from build123d import *

# Parameters (mm, degrees)
SKETCH_1_W          = 69.038205547
SKETCH_1_H          = 75.629640719
EXTRUDE_1_DEPTH     = 10
CUT_EXTRUDE_1_DEPTH = 103.8888545
FILLET_1_R          = 2
SHELL_START         = 2
SHELL_1_DEPTH       = 65.038205547
SKETCH_3_W          = 9
SKETCH_3_H          = 9
CUT_EXTRUDE_2_DEPTH = 103.887957646


# Read off the part's stored shape, not the designer's step: 쉘1
with BuildPart() as part:
    # 스케치1 → 보스-돌출1 (new body)
    with BuildSketch(Plane.XY):
        with Locations((34.519102774, 37.81482036)):
            Rectangle(SKETCH_1_W, SKETCH_1_H)
    extrude(amount=EXTRUDE_1_DEPTH)

    # 스케치2 → 컷-돌출1 (cut, through all)
    with BuildSketch(Plane(origin=(69.038205547, 0, 0), x_dir=(0, 0, -1), z_dir=(1, 0, 0))):
        with BuildLine():
            Line((-10, 75.629640719), (-10, 0))
            add(Edge.make_bspline(
                [(-5.96238454, 75.629640719), (-9.875617916, 37.91260995), (-10, 0)],
                knots=[0, 0, 0, 1, 1, 1], degree=2))
            Line((-5.96238454, 75.629640719), (-10, 75.629640719))
        make_face()
    extrude(amount=-CUT_EXTRUDE_1_DEPTH, mode=Mode.SUBTRACT)

    # 필렛1
    fillet_1_edges = [part.edges().sort_by_distance(p)[0] for p in [
        (69.038205547, 37.865383105, 8.928316045),
        (34.519102774, 75.629640719, 5.96238454),
        (0, 37.865383105, 8.928316045),
        (34.519102774, 0, 10),
    ]]
    fillet(fillet_1_edges, radius=FILLET_1_R)

    # 쉘1 outline → 쉘1 (cut)
    with BuildSketch(Plane.YZ.offset(SHELL_START)):
        with BuildLine():
            Line((73.629640719, 0), (73.62964072, 4.156994713))
            add(Edge.make_bspline(
                [(73.62964072, 4.156994713), (55.766087317, 5.967380338), (37.873438197, 7.209785835), (19.951481081, 7.884254009), (1.999999998, 7.9907666)],
                knots=[0.023838454, 0.023838454, 0.023838454, 0.023838454, 0.023838454, 0.973465237, 0.973465237, 0.973465237, 0.973465237, 0.973465237], degree=4))
            Line((1.999999998, 7.9907666), (2, 0))
            Line((2, 0), (73.629640719, 0))
        make_face()
    extrude(amount=SHELL_1_DEPTH, mode=Mode.SUBTRACT)

    # 스케치3 → 컷-돌출2 (cut, through all)
    with BuildSketch(Plane.XY):
        with Locations((18.060506117, 48.552575582)):
            Rectangle(SKETCH_3_W, SKETCH_3_H)
        with Locations((50.97769943, 48.552575582)):
            Rectangle(SKETCH_3_W, SKETCH_3_H)
    extrude(amount=CUT_EXTRUDE_2_DEPTH, mode=Mode.SUBTRACT)


solid = part.part
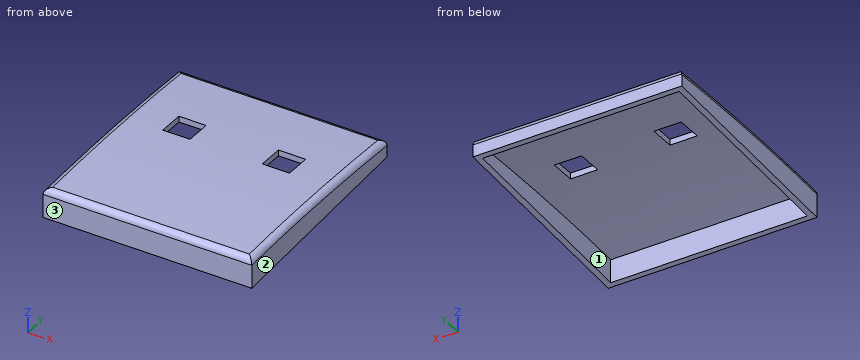
Can you work these out from the model? Positions are in its coordinate system, mm. Face numbers are marked on the shaded views. Round coordinates to 2 decimals unless told otherwise and drop trailing zeros. Order: outer loops, then holes, each group sorted by start corner. A loop starts at its lowest first (then second) coordinate and runs counter-clockwise, first axis right, second up. Notation, with made-up numbers: M -3,64.5 L 38,64.5 A27 ccw 38,88.5 Z; hole C -2,51.5 d4. An arc over 180 degrees is marked long. Use a Markdown table: item, result.
1) I'm going to push flat-ended pins straight in: P1, Ø2, axis at y = 49, z = 7.5, coming from the +X side; P2, Ø2, axis at x = 45.5, y = 11, coming from the +Z side; P3, Ø0.8, axis at y = 50.5, z = 7.5, coming from the -X side. Where does each tip first touch, or does it pass through?
Geometry says:
| item | result |
|---|---|
| P1 | stops at x = 69.02 |
| P2 | stops at z = 9.9 |
| P3 | stops at x = 0.24 |
2) Imagine slicing it at B-B (y = 47.5). Give the number of separate pieces and of enclosed holes in the cut face, then the cut area to 3 significant figures.
Geometry says:
| item | result |
|---|---|
| separate pieces | 3 |
| enclosed holes | 0 |
| area | 126 mm² |
3) If we mould it in two halves opening along Y, with no side actions, what happens to the marked faces 1, 2 and 3? For each: +Y half, -Y half, draft (parallel to the pull), parting line (faces both ways), or undercut.
Geometry says:
| item | result |
|---|---|
| face 1 | undercut |
| face 2 | draft |
| face 3 | -Y half |
4) Imagine slicing it at A-A (z = 1.5). List the corners of the cut face in (x, y) for me.
Geometry says:
| item | result |
|---|---|
| outline | M 0,0 L 69.04,0 L 69.04,75.63 L 0,75.63 Z; hole M 2,2 L 67.04,2 L 67.04,73.63 L 2,73.63 Z |
5) If I drill on line 1 along X through (y, z) = (45, 6); line 2 along Y through (x, z) = (40.5, 2.25); line 3 along X through (y, z) = (59.5, 5.5), over which ranges is the centre line in solid material (lowest first)?
Geometry says:
| item | result |
|---|---|
| line 1 | x = 0 to 2, 67.04 to 69.04 |
| line 2 | y = 0 to 2, 73.63 to 75.63 |
| line 3 | x = 0 to 69.04 |
